Source: CAD feature listing. Evaluate the final solid. Frame: model axes, mm. Face numbers are marked on the shaded views. A direction names the side the tool comes from. Give positions to 0.01 mm unless a question says otherwise; leave off trailing zeros. Order: outer loops, then holes, each group sorted by start corner. A loop starts at its lowest first (then second) coordinate and runs counter-clockwise, first axis right, second up. Notation, with made-up numbers: M -39.5,40.25 L 11.5,40.25 A30 ccw 11.5,66.25 Z; hole C -11,-3 d1. An arc over 180 degrees is marked long. Answer as a JSON object with one key per item and string values. Group by question number.
1. Pin query (flat end, axial travel): P1, Ø14.5, axis at x = 35, y = 0, coming from the -Z side; P2, Ø14.5, axis at x = 32, y = 3, coming from the +Z side; P3, Ø11, axis at y = 9, z = 29, coming from the +X side. Return the tip coordinate at first contact, or that it passes through.
2. Set-up query: the marked faces 4, 5 and 6. Return all of +Z, -Z, +X, -X, +Y, -Y with unobstructed straight access to the full face (end or side cutting, diameter ignored); none if empty.
3. Section query A-A (x = 1). Output: boundary loops of the cut face in (y, z), plus the area to 3 significant figures.
4. Section query C-C (z = 24). Output: boundary loops of the cut face in (x, y), plus the area to 3 significant figures.
5. Section query B-B (y = 14). Output: boundary loops of the cut face in (x, z), plus the area to 3 significant figures.
6. Pull-direction query (X, two-part tool) for the marked faces 1, 2 and 3; classes: +X half, -X half, draft (parallel to the pull), parting line (faces both ways), or undercut.
7. Material intervals for L1, parallel to Y at x = 2, z = -26.5; L2, parallel to Z at x = 34.5, y = 3.25; L3, parallel to X at y = -3, z = -22, sorted ascending. Write a range as [from, to].
8. Section query D-D (y = -4.75). Output: boundary loops of the cut face in (x, z).
from build123d import *

# Parameters (mm, degrees)
BOSS_EXTRUDE1_DEPTH = 38.63
BOSS_EXTRUDE2_DEPTH = 25.25
SKETCH13_W          = 26.671300946
SKETCH13_H          = 17.817336211
BOSS_EXTRUDE3_DEPTH = 77.26
BOSS_EXTRUDE4_DEPTH = 50.5
SKETCH15_W          = 43.18
SKETCH15_H          = 24.9
BOSS_EXTRUDE5_DEPTH = 77.26


with BuildPart() as part:
    # Sketch2 → Boss-Extrude1 (new body)
    with BuildSketch(Plane(origin=(0, 0, 0), x_dir=(0, 0, -1), z_dir=(1, 0, 0))):
        with BuildLine():
            Line((-8.235, -8.9), (-20.12, -8.9))
            Line((-20.12, -8.9), (-21.59, -7.43))
            Line((-21.59, -7.43), (-21.59, 14.03))
            Line((-21.59, 14.03), (-20.12, 15.5))
            Line((-20.12, 15.5), (0, 15.5))
            Line((0, 15.5), (0, 3.015))
            Line((0, 3.015), (-7.65, 3.015))
            Line((-7.65, 3.015), (-8.003553391, 2.661446609))
            ThreePointArc((-8.003553391, 2.661446609), (-8.484745674, 1.499745674), (-9.646446609, 1.018553391))
            Line((-9.646446609, 1.018553391), (-10, 0.665))
            Line((-10, 0.665), (-10, -0.665))
            Line((-10, -0.665), (-9.646446609, -1.018553391))
            ThreePointArc((-9.646446609, -1.018553391), (-8.484745674, -1.499745674), (-8.003553391, -2.661446609))
            Line((-8.003553391, -2.661446609), (-6.5, -4.165))
            Line((-6.5, -4.165), (-6.5, -7.165))
            Line((-6.5, -7.165), (-8.235, -8.9))
        make_face()
    extrude(amount=BOSS_EXTRUDE1_DEPTH)

    # Sketch3 → Boss-Extrude2 (add)
    with BuildSketch(Plane(origin=(0, 0, 0), x_dir=(0, 0, -1), z_dir=(1, 0, 0))):
        Polygon((-20.12, -8.9), (-21.12, -8.9), (-22.534213562, -7.485786438), (-26.320335651, 6.644213562), (-31.5, 6.644213562), (-31.5, 16), (-20.855, 16), (-20.855, 15.6), (-5.355, 15.6), (-5.355, 16), (0, 16), (0, 15.5), (-20.12, 15.5), (-21.59, 14.03), (-21.59, -7.43), align=None)
    extrude(amount=BOSS_EXTRUDE2_DEPTH)

    # Mirror1: part across plane


with BuildPart() as part_1:
    add(part.part)
    add(part.part.mirror(Plane.XY))

    # Mirror2: part across plane


with BuildPart() as part_2:
    add(part_1.part)
    add(part_1.part.mirror(Plane(origin=(0, 0, 0), x_dir=(0, 0, 1), z_dir=(1, 0, 0))))

    # Sketch13 → Boss-Extrude3 (add)
    with BuildSketch(Plane(origin=(38.63, 0, 0), x_dir=(0, 0, -1), z_dir=(1, 0, 0))):
        with Locations((0.075172776, 0.008668105)):
            Rectangle(SKETCH13_W, SKETCH13_H)
    extrude(amount=-BOSS_EXTRUDE3_DEPTH)

    # Sketch14 → Boss-Extrude4 (add)
    with BuildSketch(Plane(origin=(25.25, 0, 0), x_dir=(0, 0, -1), z_dir=(1, 0, 0))):
        Polygon((-31.5, 16), (31.5, 16), (31.5, 6.644213562), (26.320335651, 6.644213562), (22.15527618, -8.9), (-22.15527618, -8.9), (-26.320335651, 6.644213562), (-31.5, 6.644213562), align=None)
    extrude(amount=-BOSS_EXTRUDE4_DEPTH)

    # Sketch15 → Boss-Extrude5 (add)
    with BuildSketch(Plane(origin=(38.63, 0, 0), x_dir=(0, 0, -1), z_dir=(1, 0, 0))):
        with Locations((0, 3.55)):
            Rectangle(SKETCH15_W, SKETCH15_H)
    extrude(amount=-BOSS_EXTRUDE5_DEPTH)


solid = part_2.part
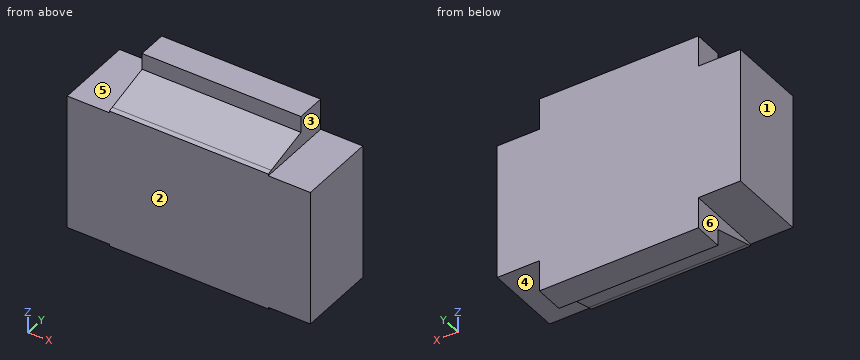
Answer sheet:
{
 "1": {"P1": "z = -21.59", "P2": "z = 26.05", "P3": "x = 25.25"},
 "2": {"face 4": "-Z, +X, +Y, -Y", "face 5": "+Z, -X, +Y, -Y", "face 6": "-Z, -X, +Y, -Y"},
 "3": {"outline": "M -8.9,-22.16 L 6.64,-26.32 L 6.64,-31.5 L 16,-31.5 L 16,31.5 L 6.64,31.5 L 6.64,26.32 L -8.9,22.16 Z", "area": "1,340 mm^2"},
 "4": {"outline": "M -25.25,-2.02 L 25.25,-2.02 L 25.25,16 L -25.25,16 Z", "area": "910 mm^2"},
 "5": {"outline": "M -38.63,-21.59 L -25.25,-21.59 L -25.25,-31.5 L 25.25,-31.5 L 25.25,-21.59 L 38.63,-21.59 L 38.63,21.59 L 25.25,21.59 L 25.25,31.5 L -25.25,31.5 L -25.25,21.59 L -38.63,21.59 Z", "area": "4,340 mm^2"},
 "6": {"face 1": "-X half", "face 2": "draft", "face 3": "+X half"},
 "7": {"L1": "[6.64, 16]", "L2": "[-21.59, 21.59]", "L3": "[-25.25, 25.25]"},
 "8": {"outline": "M -38.63,-21.59 L -25.25,-21.59 L -25.25,-23.27 L 25.25,-23.27 L 25.25,-21.59 L 38.63,-21.59 L 38.63,21.59 L 25.25,21.59 L 25.25,23.27 L -25.25,23.27 L -25.25,21.59 L -38.63,21.59 Z"}
}
